from build123d import *

# Parameters (mm, degrees)
F0_R     = 0.6093226382
F0_R_2   = 3.175
F1_DEPTH = 12.7


with BuildPart() as f1:
    # F0 (on Front) → F1 (new body)
    with BuildSketch(Plane.XZ):
        with BuildLine():
            ThreePointArc((31.5328345598, 20.6802571494), (29.770402539, 26.4681944004), (25.0812980369, 30.2916330645))
            Line((25.0812980369, 30.2916330645), (25.0812980369, 11.0688812343))
            ThreePointArc((25.0812980369, 11.0688812343), (29.770402539, 14.8923198983), (31.5328345598, 20.6802571494))
        make_face()
        with Locations((27.1492786705, 15.6318955123)):
            Circle(F0_R, mode=Mode.SUBTRACT)
        with BuildLine():
            Line((25.0812980369, 11.0688812343), (25.0812980369, 30.2916330645))
            ThreePointArc((25.0812980369, 30.2916330645), (10.7624537347, 20.6802571494), (25.0812980369, 11.0688812343))
        make_face()
        with Locations((21.1476441473, 20.6802571494)):
            Circle(F0_R_2, mode=Mode.SUBTRACT)
    extrude(amount=F1_DEPTH)


solid = f1.part
Work out the finished part from the listing and answer in its coordinate system (mm). Round coordinates to 2 decimals unless told otherwise and drop trailing zeros. Loops run counter-clockwise (first coordinate to the right, second up) from the corner with the lowest first, then second, coordinate; pieces in that order, holes last. Notation, with made-up numbers: (-18, 21.25) -> (31, 21.25) arc R27 cw to (31, 60.25) -> close; hole circle Ø9 at (-24, 16). An arc over 180 degrees is marked (long way). Use one line per item in the form item = value.
(1) Straight lines are drawn through the part: line 1 (Z direction, x = 21, y = -10.5); line 2 (Z direction, x = 19.5, y = -10.5); line 3 (X direction, y = -1, z = 21). For each, find the intervals that lie inside material, in ascending order.
Answer list:
line_1 = 10.3 to 17.51, 23.85 to 31.06
line_2 = 10.43 to 17.97, 23.39 to 30.93
line_3 = 10.77 to 17.99, 24.31 to 31.53
(2) Find section C-C on y = -8. Give the vertices of the cut face in (x, z) (3 decimals), then the cut area to 3 significant figures.
Answer list:
outline = circle Ø20.77 at (21.148, 20.68); hole circle Ø6.35 at (21.148, 20.68); hole circle Ø1.219 at (27.149, 15.632)
area = 306 mm2
(3) For a pull along X with two mould halves and no side action, classify faces 1 (the cylindrical face through (26.666, -6.261, 15.261)), 2 (the flat face through (18.7, -12.7, 23.1)) as released by +X, released by -X, zero draft, split by the parting line, or undercut.
Answer list:
face_1 = undercut
face_2 = zero draft
(4) Flat-ended cylindrical pins translate along their axes: P1, Ø3, axis at y = -2, z = 13.5, coming from the -X side; P2, Ø0.7, axis at x = 27.15, z = 15.63, coming from the +Y side; P3, Ø1, axis at x = 26.5, y = -11.5, coming from the +Z side; P4, Ø4, axis at x = 17.5, y = -2, coming from the +Z side. Find the tip coordinate at first contact, or state that the pin passes through.
Answer list:
P1 = 12.45
P2 = through
P3 = 29.86
P4 = 30.93
(5) Find section B-B on x = 23.25. Give the vertices of the cut face in (y, z).
Answer list:
outline = (-12.7, 10.51) -> (0, 10.51) -> (0, 18.3) -> (-12.7, 18.3) -> close; (-12.7, 23.06) -> (0, 23.06) -> (0, 30.85) -> (-12.7, 30.85) -> close
(6) Find section D-D on x = 16. Give the vertices of the cut face in (y, z), then the cut area to 3 significant figures.
Answer list:
outline = (-12.7, 11.66) -> (0, 11.66) -> (0, 29.7) -> (-12.7, 29.7) -> close
area = 229 mm2
(7) Find section A-A on z = 18.75. Give the vertices of the cut face in (x, y), then the cut area to 3 significant figures.
Answer list:
outline = (10.94, -12.7) -> (18.63, -12.7) -> (18.63, 0) -> (10.94, 0) -> close; (23.67, -12.7) -> (31.35, -12.7) -> (31.35, 0) -> (23.67, 0) -> close
area = 195 mm2
